from build123d import *

# Parameters (mm, degrees)
SKETCH1_W                    = 229
SKETCH1_H                    = 120
BOSS_EXTRUDE1_DEPTH          = 10
SKETCH2_W                    = 20.632503002
SKETCH2_H                    = 53.730004003
BOSS_EXTRUDE2_DEPTH          = 10
F_12_5_12_5_DIAMETER_HOLE1_D = 12.5
M6_CLEARANCE_HOLE1_D         = 6.4
F_8_0MM_DOWEL_HOLE1_D        = 8
M8_CLEARANCE_HOLE1_D         = 8.4


with BuildPart() as part:
    # Sketch1 → Boss-Extrude1 (new body)
    with BuildSketch(Plane(origin=(0, 0, 0), x_dir=(1, 0, 0), z_dir=(0, 1, 0))):
        with Locations((-114.5, 0)):
            Rectangle(SKETCH1_W, SKETCH1_H)
    extrude(amount=-BOSS_EXTRUDE1_DEPTH)

    # Sketch2 → Boss-Extrude2 (add)
    with BuildSketch(Plane(origin=(0, 0, 0), x_dir=(1, 0, 0), z_dir=(0, 1, 0))):
        with Locations((10.316251501, 33.134997999)):
            Rectangle(SKETCH2_W, SKETCH2_H)
    extrude(amount=-BOSS_EXTRUDE2_DEPTH)

    # Ø12.5 (12.5) Diameter Hole1 (through all)
    with Locations(Plane(origin=(0, -10, 0), x_dir=(-1, 0, 0), z_dir=(0, -1, 0))):
        with Locations((9.969, 50), (79.812013925, 50.183768679), (149.323, 50), (219, 50), (219, -50), (149.323, -50), (79.646, -50), (9.969, -50)):
            Hole(F_12_5_12_5_DIAMETER_HOLE1_D / 2)

    # M6 Clearance Hole1 (through all)
    with Locations(Plane(origin=(0, -10, 0), x_dir=(-1, 0, 0), z_dir=(0, -1, 0))):
        with Locations((-2.125, 25.691000385), (39.875, 25.691000385), (77.875, 17.152366083), (119.875, 17.152366083), (157.875, 16.78), (199.875, 16.78)):
            Hole(M6_CLEARANCE_HOLE1_D / 2)

    # Ø8.0mm Dowel Hole1 (through all)
    with Locations(Plane(origin=(0, -10, 0), x_dir=(-1, 0, 0), z_dir=(0, -1, 0))):
        with Locations((184.75, -48), (44.219, 48)):
            Hole(F_8_0MM_DOWEL_HOLE1_D / 2)

    # M8 Clearance Hole1 (through all)
    with Locations(Plane(origin=(0, -10, 0), x_dir=(-1, 0, 0), z_dir=(0, -1, 0))):
        with Locations((28.219, 48), (200.75, 48), (200.75, -48), (28.219, -48)):
            Hole(M8_CLEARANCE_HOLE1_D / 2)


solid = part.part
Geometry: final body of the model. Coordinates: model frame, mm. A direction names the side the tool comes from. Round coordinates to 2 decimals unless told otherwise and drop trailing zeros. Loops run counter-clockwise (first coordinate to the right, second up) from the corner with the lowest first, then second, coordinate; pieces in that order, holes last. Notation, with made-up numbers: (44, -28.5) -> (66, -28.5) arc R27 cw to (66, -6.5) -> close; hole circle Ø2 at (55.25, 69.5). An arc over 180 degrees is marked (long way). One line per question, with ' | ' between items. Start each with the question number.
1. Line query: line 1 along Z through (x, y) = (-219, -6.25); line 2 along X through (y, z) = (-7.25, -16.78) (1 decimal); line 3 along Z through (x, y) = (-215.5, -3.25). Output: solid intervals per line, ascending. Write a range as [from, to].
2. Section A-A on x = -219. Output: boundary loops of the cut face in (y, z), and give its area (3 significant figures).
3. Section D-D on y = -7.25. Count the separate pieces of the cut face and the enclosed holes in it, and give its area (3 significant figures).
4. Set-up query: faces 1 (the face through (10, -5, -6.27)), 2 (the face through (-154.823, -4.93, -17.741)). Return all of +Z, -Z, +X, -X, +Y, -Y with unobstructed straight access to the full face (end or side cutting, diameter ignored); none if empty.
5. Contact query for a flat-ended pin moving along its axis: pin 1 (6.5 mm diameter, centred on x = -184.75, z = 48, fed in from +Y). Output: stop coordinate, or through.
6. Mould query, pull axis X, two halves, no side actions, for faces 3 (the face through (0, -5, 27)), 4 (the face through (-223.61, -4.93, 45.78)), 5 (the face through (-106, -10, -1)). Classes: pulls with the +X half, pulls with the -X half, needs draft (parallel to the pull), parting line crosses it, or undercut.
7. Section B-B on x = -184.75. Output: boundary loops of the cut face in (y, z).
8. Section C-C on z = -4. Output: boundary loops of the cut face in (x, y), and give its area (3 significant figures).
Returned:
1) line 1: z = [-60, -56.25], [-43.75, 43.75], [56.25, 60] | line 2: x = [-229, -203.1], [-196.7, -161.1], [-154.7, -123.1], [-116.7, -81.1], [-74.7, 20.6] | line 3: z = [-60, -55.18], [-44.82, 44.82], [55.18, 60]
2) outline: (-10, -60) -> (0, -60) -> (0, -56.25) -> (-10, -56.25) -> close; (-10, -43.75) -> (0, -43.75) -> (0, 43.75) -> (-10, 43.75) -> close; (-10, 56.25) -> (0, 56.25) -> (0, 60) -> (-10, 60) -> close | area: 950 mm2
3) separate pieces: 1 | enclosed holes: 20 | area: 27,100 mm2
4) face 1: +Z, +X, +Y, -Y | face 2: +Y, -Y
5) pin 1: passes through
6) face 3: pulls with the +X half | face 4: undercut | face 5: needs draft
7) outline: (-10, -60) -> (0, -60) -> (0, 44) -> (-10, 44) -> close; (-10, 52) -> (0, 52) -> (0, 60) -> (-10, 60) -> close
8) outline: (-229, -10) -> (0, -10) -> (0, 0) -> (-229, 0) -> close | area: 2,290 mm2
